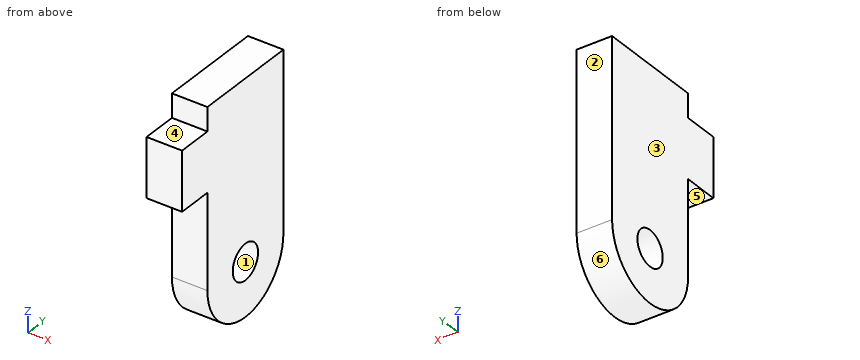
Autodesk Inventor part; units mm, degrees
ref_plane "YZ Plane" through (0, 0, 0) normal (1, 0, 0) x (0, 1, 0)
ref_plane "XZ Plane" through (0, 0, 0) normal (0, 1, 0) x (-1, 0, 0)
ref_plane "XY Plane" through (0, 0, 0) normal (0, 0, 1) x (1, 0, 0)
sketch "Sketch1" plane through (0, 0, 0) normal (1, 0, 0) x (0, 1, 0)
  line L0 (-4.5, 7.5) -> (4.5, 7.5)
  line L1 (4.5, 7.5) -> (4.5, -7.5)
  line L2 (4.5, -7.5) -> (-4.5, -7.5)
  line L3 (-4.5, -7.5) -> (-4.5, 7.5)
  line L4 (-4.5, 7.5) -> (4.5, -7.5) construction
  line L5 (4.5, 7.5) -> (-4.5, -7.5) construction
  circle A0 centre (0, -7.5) radius 4.5
  point P0 (0, 0)
  dimension "d0" = 9
  dimension "d1" = 15
  dimension "d2" = 9
extrude "Extrusion1" add sketch "Sketch1" along normal blind 3
sketch "Sketch2" plane through (0, 0, 0) normal (-1, 0, 0) x (0, 0, 1)
  arc A0 (-7.5, 4.5) -> (-7.5, -4.5) centre (-7.5, 0) ccw
  circle A1 centre (-7.5, 0) radius 1.5
  point P0 (0, 0)
  dimension "d5" = 3
extrude "Extrusion2" cut sketch "Sketch2" against normal blind 10
sketch "Sketch3" plane through (0, 0, 0) normal (-1, 0, 0) x (0, 0, 1)
  line L0 (7.5, -4.5) -> (-7.5, -4.5)
  line L1 (0.5, -4.5) -> (5.5, -4.5)
  line L2 (5.5, -4.5) -> (5.5, -7.5)
  line L3 (5.5, -7.5) -> (0.5, -7.5)
  line L4 (0.5, -7.5) -> (0.5, -4.5)
  circle A0 centre (-7.5, 0) radius 1.5
  point P0 (0, 0)
  dimension "d8" = 5
  dimension "d9" = 3
  dimension "d10" = 8
extrude "Extrusion3" add sketch "Sketch3" against normal blind 3 contours L2 L3 L4 L0
properties part number "Battey latch"
Can you work these out from the model? Positions are in its coordinate system, mm. Face numbers are marked on the shaded views. A direction names the side the tool comes from. Round coordinates to 2 decimals unless told otherwise and drop trailing zeros. Loops run counter-clockwise (first coordinate to the right, second up) from the corner with the lowest first, then second, coordinate; pieces in that order, holes last. Notation, with made-up numbers: (-15, -30.5) - (2, -30.5) arc R17 cw to (2, -24.5) - close; hole circle Ø10 at (85.25, 29.5). An arc over 180 degrees is marked (long way). Use CSV: the item, a comma, the result in double quotes. Start each with the question number.
1) If we section it at D-D on y = -4: Write out the boundary of the cut face in (x, z).
2) For pin 1 Ø0.6 at (x, z) = (1, 6) entering from -Y; pin 2 Ø1.5 at (x, y) = (1, -6.5) entering from +Z, each with a flat end and sliding along its axis, tell me the tip position at first contact or that it passes through.
3) If we section it at A-A on y = 0: Write out the boundary of the cut face in (x, z).
4) For the marked faces 4, 5 and 6, which set-ups out of +Z, -Z, +X, -X, +Y, -Y let a thin tool reach every point of the face, with its end or its side?
5) Please list where these lines run through material, in increasing order: probe 1 along Y at (x, z) = (1.3, -7.5); probe 2 along Y at (x, z) = (2.85, -2.5); probe 3 along Z at (x, y) = (1.95, -5.75). Write a range as [from, to].
6) If we section it at B-B on x = 1.55: Write out the boundary of the cut face in (y, z).
7) If we section it at C-C on z = -3.25: Write out the boundary of the cut face in (x, y).
8) We'd pull the mould along Y, two halves only. Please class the marked faces 1, 2 and 3: released by +Y, released by -Y, zero draft, split by the parting line, or undercut.
Geometry results:
1,outline,"(0, -9.56) - (3, -9.56) - (3, 7.5) - (0, 7.5) - close"
2,pin 1,"stops at y = -4.5"
2,pin 2,"stops at z = 5.5"
3,outline,"(0, -12) - (3, -12) - (3, -9) - (0, -9) - close; (0, -6) - (3, -6) - (3, 7.5) - (0, 7.5) - close"
4,face 4,"+Z, +X, -X, -Y"
4,face 5,"-Z, +X, -X, -Y"
4,face 6,"-Z, +X, -X"
5,probe 1,"y = [-4.5, -1.5], [1.5, 4.5]"
5,probe 2,"y = [-4.5, 4.5]"
5,probe 3,"z = [0.5, 5.5]"
6,outline,"(-7.5, 0.5) - (-4.5, 0.5) - (-4.5, -7.5) arc R4.5 ccw to (4.5, -7.5) - (4.5, 7.5) - (-4.5, 7.5) - (-4.5, 5.5) - (-7.5, 5.5) - close; hole circle Ø3 at (0, -7.5)"
7,outline,"(0, -4.5) - (3, -4.5) - (3, 4.5) - (0, 4.5) - close"
8,face 1,"undercut"
8,face 2,"released by +Y"
8,face 3,"zero draft"
